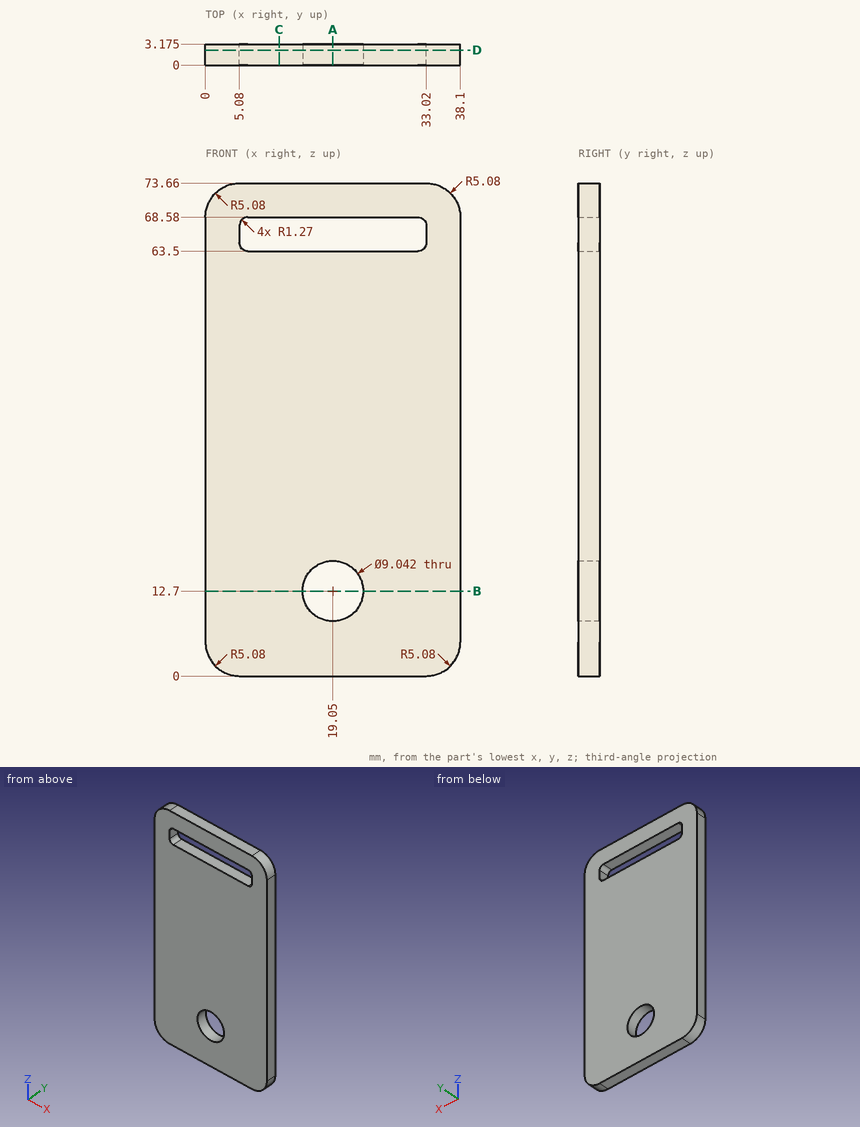
Geometry check sheet. Reference: drawing and pictorial views, mm from the part's lowest x, y, z. Coordinates: 2 decimals unless noted, no trailing zeros. Order: outer loops, then holes, each group sorted by start corner. A loop starts at its lowest first (then second) coordinate and runs counter-clockwise, first axis right, second up. Notation, with made-up numbers: (-9.75, 34.5) - (22.25, 34.5) arc R25 ccw to (22.25, 60.5) - close; hole circle Ø2 at (6.25, 19.5). An arc over 180 degrees is marked (long way). Answer in a Markdown table with one row per item. Add a question column.
1) Material ranges on line 1 along X through (y, z) = (2.45, 12.7); line 2 along Z through (x, y) = (29, 1); line 3 along Z through (x, y) = (16.5, 2.6) (1 decimal), recorded low to high. Write a range as [from, to].
2) Cross-section at A-A, the plane x = 19.05. Record the cut outline in (y, z) (1 decimal).
3) Cross-section at B-B, the plane z = 12.7. Record the cut outline in (x, y) (1 decimal).
4) Cross-section at D-D, the plane y = 2.25. Record the cut outline in (x, z), then the cut area to 3 significant figures.
5) Cross-section at C-C, the plane x = 11. Record the cut outline in (y, z) (1 decimal), then the cut area to 3 significant figures.
6) Gauge pin test, flat end, axial feed: P1, Ø7, axis at x = 19.05, z = 12.7, coming from the +Y side. Record the tip position at first contact, or that the pin passes through.
Check result:
| question | item | result |
|---|---|---|
| 1 | line 1 | x = [0, 14.53], [23.57, 38.1] |
| 1 | line 2 | z = [0, 63.5], [68.58, 73.66] |
| 1 | line 3 | z = [0, 9], [16.4, 63.5], [68.6, 73.7] |
| 2 | outline | (0, 0) - (3.2, 0) - (3.2, 8.2) - (0, 8.2) - close; (0, 17.2) - (3.2, 17.2) - (3.2, 63.5) - (0, 63.5) - close; (0, 68.6) - (3.2, 68.6) - (3.2, 73.7) - (0, 73.7) - close |
| 3 | outline | (0, 0) - (14.5, 0) - (14.5, 3.2) - (0, 3.2) - close; (23.6, 0) - (38.1, 0) - (38.1, 3.2) - (23.6, 3.2) - close |
| 4 | outline | (0, 5.08) arc R5.08 ccw to (5.08, 0) - (33.02, 0) arc R5.08 ccw to (38.1, 5.08) - (38.1, 68.58) arc R5.08 ccw to (33.02, 73.66) - (5.08, 73.66) arc R5.08 ccw to (0, 68.58) - close; hole (5.08, 64.77) arc R1.27 ccw to (6.35, 63.5) - (31.75, 63.5) arc R1.27 ccw to (33.02, 64.77) - (33.02, 67.31) arc R1.27 ccw to (31.75, 68.58) - (6.35, 68.58) arc R1.27 ccw to (5.08, 67.31) - close; hole circle Ø9.04 at (19.05, 12.7) |
| 4 | area | 2,580 mm² |
| 5 | outline | (0, 0) - (3.2, 0) - (3.2, 63.5) - (0, 63.5) - close; (0, 68.6) - (3.2, 68.6) - (3.2, 73.7) - (0, 73.7) - close |
| 5 | area | 218 mm² |
| 6 | P1 | passes through |
